from build123d import *

# Parameters (mm, degrees)
CROQUIS1_R              = 1.5
SALIENTE_EXTRUIR1_DEPTH = 3


with BuildPart() as part:
    # Croquis1 → Saliente-Extruir1 (new body)
    with BuildSketch(Plane.XY):
        with BuildLine():
            Line((0, -11.947743298), (77.78, -11.947743298))
            ThreePointArc((77.78, -11.947743298), (89.727743298, 0), (77.78, 11.947743298))
            ThreePointArc((77.78, 11.947743298), (38.89, 40.683911684), (0, 11.947743298))
            ThreePointArc((0, 11.947743298), (-11.947743298, 0), (0, -11.947743298))
        make_face()
        Circle(CROQUIS1_R, mode=Mode.SUBTRACT)
        with Locations((77.78, 0)):
            Circle(CROQUIS1_R, mode=Mode.SUBTRACT)
        with Locations((38.89, 30)):
            Circle(CROQUIS1_R, mode=Mode.SUBTRACT)
    extrude(amount=SALIENTE_EXTRUIR1_DEPTH)


solid = part.part
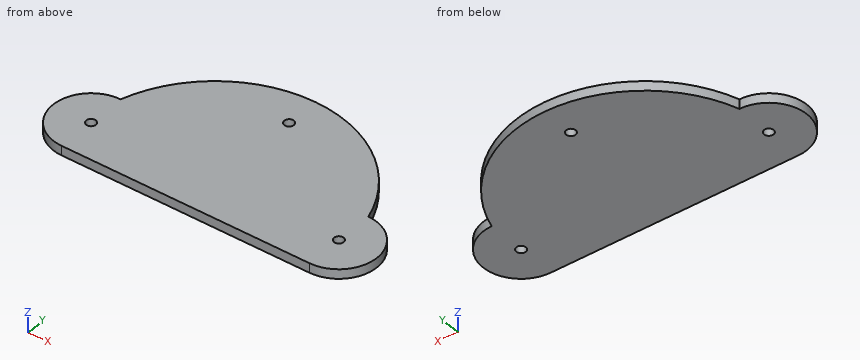
Verification items for the finished model (mm, model axes). Coordinates: 2 decimals unless noted, no trailing zeros. Loops run counter-clockwise (first coordinate to the right, second up) from the corner with the lowest first, then second, coordinate; pieces in that order, holes last. Notation, with made-up numbers: (-22.75, -31.5) -> (9.25, -31.5) arc R6 cw to (9.25, -22.5) -> close; hole circle Ø6 at (82.5, 27.25). An arc over 180 degrees is marked (long way). Write each question's results on one line, items separated by ' | '.
Item 1: Section check C-C, the plane y = 0. Enter the section's corners in (x, z).
Found:
outline: (-11.95, 0) -> (-1.5, 0) -> (-1.5, 3) -> (-11.95, 3) -> close; (1.5, 0) -> (76.28, 0) -> (76.28, 3) -> (1.5, 3) -> close; (79.28, 0) -> (89.73, 0) -> (89.73, 3) -> (79.28, 3) -> close
Item 2: Section check B-B, the plane x = 38.89. Enter the section's corners in (y, z).
Found:
outline: (-11.95, 0) -> (28.5, 0) -> (28.5, 3) -> (-11.95, 3) -> close; (31.5, 0) -> (40.68, 0) -> (40.68, 3) -> (31.5, 3) -> close
Item 3: Section check A-A, the plane z = 1.25. Enter the section's corners in (x, y).
Found:
outline: (0, -11.95) -> (77.78, -11.95) arc R11.95 ccw to (77.78, 11.95) arc R40.68 ccw to (0, 11.95) arc R11.95 ccw to start; hole circle Ø3 at (0, 0); hole circle Ø3 at (38.89, 30); hole circle Ø3 at (77.78, 0)
Item 4: Section check D-D, the plane y = -6. Enter the section's corners in (x, z).
Found:
outline: (-10.33, 0) -> (88.11, 0) -> (88.11, 3) -> (-10.33, 3) -> close
Item 5: Gauge pin test, flat end, axial feed: pin 1 (2.5 mm diameter, centred on x = 38.89, y = 30, fed in from -Z). Record the tip position at first contact, or that the pin passes through.
Found:
pin 1: passes through
Item 6: Material ranges on L1, parallel to X at y = 0.5, z = 1.5; L2, parallel to Y at x = 38.89, z = 2.3; L3, parallel to Y at x = 40, z = 2.25, recorded low to high.
Found:
L1: x = -11.94 to -1.41, 1.41 to 76.37, 79.19 to 89.72 | L2: y = -11.95 to 28.5, 31.5 to 40.68 | L3: y = -11.95 to 28.99, 31.01 to 40.67
